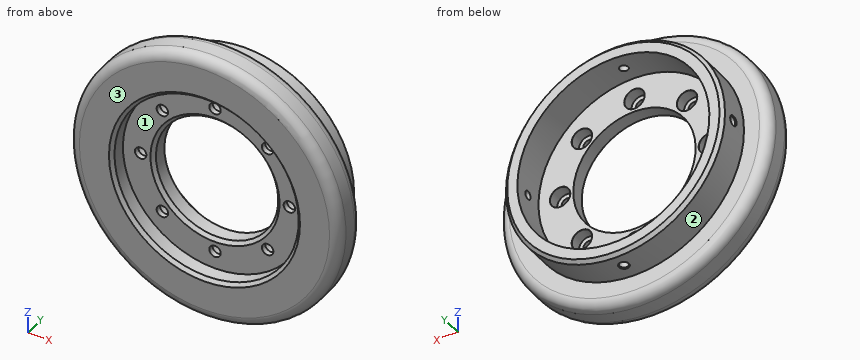
```python
from build123d import *

# Parameters (mm, degrees)
SKETCH_1_R               = 40
EXTRUDE_1_DEPTH          = 10
SKETCH_2_R               = 27.25
CUT_EXTRUDE_1_DEPTH      = 5
SKETCH_4_R               = 32.4
SKETCH_4_R_2             = 28.4
EXTRUDE_2_DEPTH          = 10
SKETCH_5_R               = 18.1
CUT_EXTRUDE_2_DEPTH      = 58.445626465
PATTERN_CIRCULAR_1_COUNT = 8
PATTERN_CIRCULAR_2_COUNT = 4
CHAMFER_1_SIZE           = 1
CHAMFER_2_SIZE           = 1
FILLET_1_R               = 3
CHAMFER_3_SIZE           = 1


# Read off the part's stored shape, not the designer's step: M3 螺纹孔1
with BuildPart() as part:
    # 草图1 → 凸台-拉伸1 (new body)
    with BuildSketch(Plane(origin=(0, 0, 0), x_dir=(1, 0, 0), z_dir=(0, 1, 0))):
        with Locations(Location((0, 0, 0), (0, 0, 270))):
            Circle(SKETCH_1_R)
    extrude(amount=EXTRUDE_1_DEPTH)

    # 草图2 → 切除-拉伸1 (cut)
    with BuildSketch(Plane.XZ):
        with Locations(Location((0, 0, 0), (0, 0, 270))):
            Circle(SKETCH_2_R)
    extrude(amount=-CUT_EXTRUDE_1_DEPTH, mode=Mode.SUBTRACT)

    # 草图4 → 凸台-拉伸2 (add)
    with BuildSketch(Plane(origin=(0, 10, 0), x_dir=(1, 0, 0), z_dir=(0, 1, 0))):
        with Locations(Location((0, 0, 0), (0, 0, 270))):
            Circle(SKETCH_4_R)
        with Locations(Location((0, 0, 0), (0, 0, 270))):
            Circle(SKETCH_4_R_2, mode=Mode.SUBTRACT)
    extrude(amount=EXTRUDE_2_DEPTH)

    # 草图5 → 切除-拉伸2 (cut, through all)
    with BuildSketch(Plane(origin=(0, 10, 0), x_dir=(1, 0, 0), z_dir=(0, 1, 0))):
        with Locations(Location((0, 0, 0), (0, 0, 270))):
            Circle(SKETCH_5_R)
    extrude(amount=-CUT_EXTRUDE_2_DEPTH, mode=Mode.SUBTRACT)

    # 草图12 → 打孔尺寸(%根据)内六角圆柱头螺钉的类型3 (revolve, cut)
    with BuildSketch(Plane(origin=(0, 10, -22), x_dir=(0, 0, 1), z_dir=(1, 0, 0))):
        Polygon((0, 0), (0, 10), (1.7, 10), (1.7, 3.4), (3, 3.4), (3, 0.025), (3.025, 0), align=None)
    hole_wizard_3 = revolve(axis=Axis((0, 16.35, -22), (0, -1, 0)), mode=Mode.SUBTRACT)

    # 阵列(圆周)1: 打孔尺寸(%根据)内六角圆柱头螺钉的类型3 ×8 about axis
    pattern_circular_1_axis = Axis((0, 0, 0), (0, 1, 0))
    for i in range(1, PATTERN_CIRCULAR_1_COUNT):
        add(hole_wizard_3.rotate(pattern_circular_1_axis, i * 360 / PATTERN_CIRCULAR_1_COUNT), mode=Mode.SUBTRACT)

    # M3 螺纹孔1 outline → M3 螺纹孔1 (revolve, cut)
    with BuildSketch(Plane(origin=(0, 15, 0), x_dir=(0, 1, 0), z_dir=(0, 0, -1))):
        Polygon((0, -32.400010655), (1.525010655, -32.400010655), (1.25, -32.125), (1.25, -28.372463058), (0, -28.372463058), align=None)
    hole_wizard_m3_1 = revolve(axis=Axis((0, 15, 0), (1, 0, 0)), mode=Mode.SUBTRACT)

    # 阵列(圆周)2: M3 螺纹孔1 ×4 about axis
    pattern_circular_2_axis = Axis((0, 20, 0), (0, -1, 0))
    for i in range(1, PATTERN_CIRCULAR_2_COUNT):
        add(hole_wizard_m3_1.rotate(pattern_circular_2_axis, i * 360 / PATTERN_CIRCULAR_2_COUNT), mode=Mode.SUBTRACT)

    # 倒角1
    chamfer_1_edges = [part.edges().sort_by_distance(p)[0] for p in [
        (0, 20, -32.4),
    ]]
    chamfer(chamfer_1_edges, length=CHAMFER_1_SIZE)

    # 倒角2
    chamfer_2_edges = [part.edges().sort_by_distance(p)[0] for p in [
        (0, 0, 27.25),
    ]]
    chamfer(chamfer_2_edges, length=CHAMFER_2_SIZE)

    # 圆角1
    fillet_1_edges = [part.edges().sort_by_distance(p)[0] for p in [
        (0, 0, -40),
        (0, 10, -40),
    ]]
    fillet(fillet_1_edges, radius=FILLET_1_R)

    # 倒角3
    chamfer_3_edges = [part.edges().sort_by_distance(p)[0] for p in [
        (0, 5, -18.1),
    ]]
    chamfer(chamfer_3_edges, length=CHAMFER_3_SIZE)


solid = part.part
```
Can you work these out from the model? Positions are in its coordinate system, mm. Face numbers are marked on the shaded views. Give positions to 0.01 mm unless a question says otherwise; leave off trailing zeros. Write each loop counter-clockwise with the first axis right and the second up, starting at its lowest first coordinate (ties: lowest second). Pieces come first, ordered by that corner, then holes. Notation, with made-up numbers: (46.5, -40) - (57.5, -40) arc R19 cw to (57.5, -5) - close; hole circle Ø11 at (18, 64). An arc over 180 degrees is marked (long way). Write item = value, one per line. Start each with the question number.
1. For pin 1 (3 mm diameter, centred on x = 14.5, z = 15.5, fed in from +Y); pin 2 (6.5 mm diameter, centred on x = 15, z = -16, fed in from +Y); pin 3 (3 mm diameter, centred on x = 0, z = -22, fed in from +Y); pin 4 (1.5 mm diameter, centred on x = 6.5, y = 10, fed in from +Z), each with a flat end and sliding along its axis, tell me the tip position at first contact or that it passes through.
2. Imagine slicing it at B-B (y = 9). Count the separate pieces of the cut face and the enclosed holes in it, and give its area (3 significant figures).
3. Please list where these lines run through material, in increasing order: line 1 (Z direction, x = -1, y = 12.5); line 2 (Y direction, x = -26.5, z = -2); line 3 (Z direction, x = 23, y = 12.5).
4. Thinking about a two-plate mould opening in Z: for the marked faces 1, 2 and 3, which applies, released by +Z, released by -Z, zero draft, split by the parting line, or undercut?
5. Imagine slicing it at A-A (y = 15). Please give me the cut outline in (x, z) (3 decimals).
Worked answers:
q1.pin_1 = 6.6
q1.pin_2 = 10
q1.pin_3 = through
q1.pin_4 = 38.45
q2.separate_pieces = 1
q2.enclosed_holes = 9
q2.area = 3,580 mm2
q3.line_1 = -32.38 to -28.38, 28.38 to 32.38
q3.line_2 = 5 to 10
q3.line_3 = -22.82 to -16.66, 16.66 to 22.82
q4.face_1 = undercut
q4.face_2 = split by the parting line
q4.face_3 = zero draft
q5.outline = (-32.366, -1.491) arc R32.4 ccw to (-1.491, -32.366) - (-1.25, -32.125) - (-1.25, -28.372) arc R28.4 cw to (-28.372, -1.25) - (-32.125, -1.25) - close; (-32.366, 1.491) - (-32.125, 1.25) - (-28.372, 1.25) arc R28.4 cw to (-1.25, 28.372) - (-1.25, 32.125) - (-1.491, 32.366) arc R32.4 ccw to start; (1.25, -32.125) - (1.491, -32.366) arc R32.4 ccw to (32.366, -1.491) - (32.125, -1.25) - (28.372, -1.25) arc R28.4 cw to (1.25, -28.372) - close; (1.25, 28.372) arc R28.4 cw to (28.372, 1.25) - (32.125, 1.25) - (32.366, 1.491) arc R32.4 ccw to (1.491, 32.366) - (1.25, 32.125) - close
